Build history of the part. All positions in model axes, mm. Round coordinates to 2 decimals unless told otherwise and drop trailing zeros. Write each loop counter-clockwise with the first axis right and the second up, starting at its lowest first coordinate (ties: lowest second). Pieces come first, ordered by that corner, then holes. Notation, with made-up numbers: M 68.25,37.5 L 96.25,37.5 A35 cw 96.25,70.5 Z; hole C 58.5,-27 d11. An arc over 180 degrees is marked long. Use a Markdown table: item, result.
from build123d import *

# Parameters (mm, degrees)
SKETCH1_R           = 12.5
BOSS_EXTRUDE1_DEPTH = 2
SKETCH2_R           = 3.7
BOSS_EXTRUDE2_DEPTH = 3


with BuildPart() as part:
    # Sketch1 → Boss-Extrude1 (new body)
    with BuildSketch(Plane(origin=(0, 0, 0), x_dir=(1, 0, 0), z_dir=(0, 1, 0))):
        Circle(SKETCH1_R)
        with BuildLine():
            Line((1.095445115, -1.3), (-1.095445115, -1.3))
            ThreePointArc((-1.095445115, -1.3), (0, 1.7), (1.095445115, -1.3))
        make_face(mode=Mode.SUBTRACT)
    extrude(amount=BOSS_EXTRUDE1_DEPTH)

    # Sketch2 → Boss-Extrude2 (add)
    with BuildSketch(Plane(origin=(0, 2, 0), x_dir=(1, 0, 0), z_dir=(0, 1, 0))):
        Circle(SKETCH2_R)
        with BuildLine():
            Line((-1.095445115, -1.3), (1.095445115, -1.3))
            ThreePointArc((1.095445115, -1.3), (0, 1.7), (-1.095445115, -1.3))
        make_face(mode=Mode.SUBTRACT)
    extrude(amount=BOSS_EXTRUDE2_DEPTH)


solid = part.part
Q1. Cut at B-B on x = 0. Give the cut face in (y, z), and give its area (3 significant figures).
Response values:
| item | result |
|---|---|
| outline | M 0,-12.5 L 2,-12.5 L 2,-3.7 L 5,-3.7 L 5,-1.7 L 0,-1.7 Z; M 0,1.3 L 5,1.3 L 5,3.7 L 2,3.7 L 2,12.5 L 0,12.5 Z |
| area | 57.2 mm2 |
Q2. Cut at C-C on y = 2.65. Give the cut face in (x, z).
Response values:
| item | result |
|---|---|
| outline | C 0,0 d7.4; hole M -1.1,1.3 A1.7 ccw long 1.1,1.3 Z |
Q3. Cut at A-A on z = 0. Give the cut face in (x, y).
Response values:
| item | result |
|---|---|
| outline | M -12.5,0 L -1.7,0 L -1.7,5 L -3.7,5 L -3.7,2 L -12.5,2 Z; M 1.7,0 L 12.5,0 L 12.5,2 L 3.7,2 L 3.7,5 L 1.7,5 Z |
Q4. Drop flat-ended pins along their axis: P1, Ø0.7, axis at x = 0, y = 2.5, coming from the -Z side; P2, Ø2, axis at x = -7, y = 1, coming from the +Z side. Give the stop position or say it passes through.
Response values:
| item | result |
|---|---|
| P1 | stops at z = -3.7 |
| P2 | stops at z = 10.97 |
Q5. Drill centre lines: L1, parallel to X at y = 1.1, z = 0; L2, parallel to Z at x = 0, y = 2.7; L3, parallel to X at y = 3.2, z = 0. Where is each one in solid material? Low to high.
Response values:
| item | result |
|---|---|
| L1 | x = -12.5 to -1.7, 1.7 to 12.5 |
| L2 | z = -3.7 to -1.7, 1.3 to 3.7 |
| L3 | x = -3.7 to -1.7, 1.7 to 3.7 |
Q6. Cut at D-D on z = 7.5. Give the cut face in (x, y), and give its area (3 significant figures).
Response values:
| item | result |
|---|---|
| outline | M -10,0 L 10,0 L 10,2 L -10,2 Z |
| area | 40.0 mm2 |
Q7. Two-plate mould, pull along Z, no slides. Class faces 1 (the cylindrical face through (-0.802, 3.479, 3.612)), 2 (the flat face through (0, 2, 1.3)), 3 (the flat face through (-3, 2, 3)): +Z half, -Z half, draft (parallel to the pull), parting line (faces both ways), or undercut.
Response values:
| item | result |
|---|---|
| face 1 | parting line |
| face 2 | undercut |
| face 3 | draft |
